Check sheet for the modelled part. Datum: model origin and axes. Units: mm. Coordinates: 2 decimals unless noted, no trailing zeros. Order: outer loops, then holes, each group sorted by start corner. A loop starts at its lowest first (then second) coordinate and runs counter-clockwise, first axis right, second up.
from build123d import *

# Parameters (mm, degrees)
BOSS_EXTRUDE2_DEPTH = 25.62


with BuildPart() as part:
    # Sketch3 → Boss-Extrude2 (new body)
    with BuildSketch(Plane(origin=(0, 0, 0), x_dir=(1, 0, 0), z_dir=(0, 1, 0))):
        with BuildLine():
            ThreePointArc((-4.193822504, 6.7), (-4.397207794, 4.397207794), (-6.7, 4.193822504))
            Line((-6.7, 4.193822504), (-6.7, 3.87))
            Line((-6.7, 3.87), (-6.7, -3.87))
            Line((-6.7, -3.87), (-7.47, -3.87))
            Line((-7.47, -3.87), (-7.47, 3.87))
            Line((-7.47, 3.87), (-7.47, 5.67))
            ThreePointArc((-7.47, 5.67), (-6.942792206, 6.942792206), (-5.67, 7.47))
            Line((-5.67, 7.47), (-3.87, 7.47))
            Line((-3.87, 7.47), (3.87, 7.47))
            Line((3.87, 7.47), (3.87, 6.7))
            Line((3.87, 6.7), (-3.87, 6.7))
            Line((-3.87, 6.7), (-4.193822504, 6.7))
        make_face()
    extrude(amount=BOSS_EXTRUDE2_DEPTH)


solid = part.part
(1) Cross-section at C-C (x = -1.5). Enter the section's corners in (y, z), and give its area (3 significant figures).
Filled in:
outline: (0, -7.47) - (25.62, -7.47) - (25.62, -6.7) - (0, -6.7) - close
area: 19.7 mm2
(2) Thickness scan on probe 1 along Z at (x, y) = (-1, 19.5); probe 2 along X at (y, z) = (9.25, -5.75). Record the ranges inside material, lowest first.
Filled in:
probe 1: z = -7.47 to -6.7
probe 2: x = -7.47 to -3.87
(3) Release check for a two-part mould opening along Z. For faces 1 (the cylindrical face through (-6.957, 12.631, -6.929)), 2 (the flat face through (-4.71, 25.62, -4.35)), 3 (the cylindrical face through (-4.373, 12.631, -4.422)) record: +Z half, -Z half, draft (parallel to the pull), parting line (faces both ways), or undercut.
Filled in:
face 1: -Z half
face 2: draft
face 3: undercut
(4) Cross-section at B-B (z = 0). Enter the section's corners in (x, y).
Filled in:
outline: (-7.47, 0) - (-6.7, 0) - (-6.7, 25.62) - (-7.47, 25.62) - close
(5) Go/stop test with flat-tipped pins: P1, Ø6.5, axis at y = 18, z = 0.5, coming from the +X side; P2, Ø5, axis at x = 0, z = -2.5, coming from the -Y side. Record where each tip stops, or that it passes through.
Filled in:
P1: stops at x = -6.7
P2: passes through
(6) Cross-section at A-A (y = 4.5). Enter the section's corners in (x, z), and give its area (3 significant figures).
Filled in:
outline: (-7.47, -5.67) arc R1.8 ccw to (-5.67, -7.47) - (3.87, -7.47) - (3.87, -6.7) - (-4.19, -6.7) arc R1.8 ccw to (-6.7, -4.19) - (-6.7, 3.87) - (-7.47, 3.87) - close
area: 23.3 mm2
